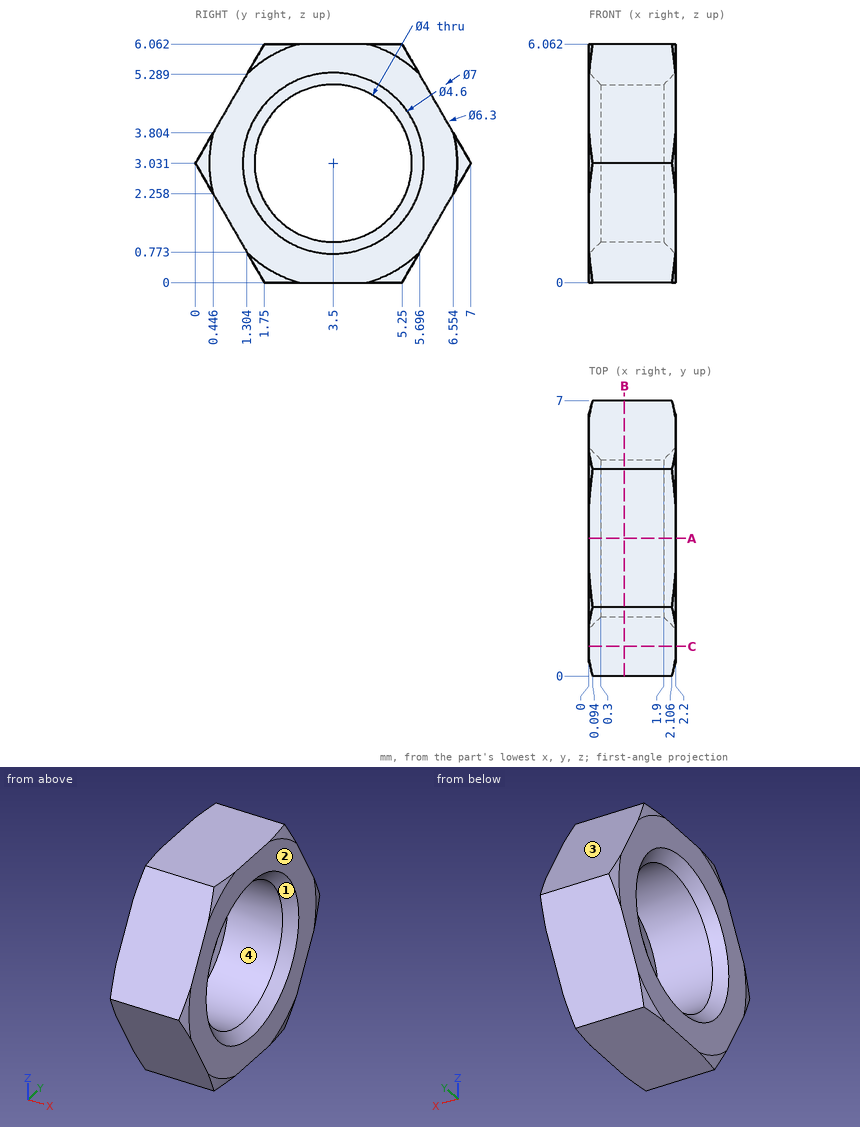
Answer from the drawing. Dimensions are ordinates in mm from the lowest x, y and z of the part. Give positions to 0.01 mm unless a question says otherwise; leave off trailing zeros. Write each loop counter-clockwise with the first axis right and the second up, starting at its lowest first coordinate (ties: lowest second). Pieces come first, ordered by that corner, then holes. Notation, with made-up numbers: M 58.25,50 L 86.25,50 A9 ccw 86.25,63 Z; hole C -9.5,65.25 d5. An arc over 180 degrees is marked long. Answer as CSV lines item,"result".
Q1. Given P1, Ø1.5, axis at y = 1, z = 3.5, coming from the -X side, flat-ended and moving along its own axis, determine where the tip first touches the part or whether it passes through.
A:
P1,"stops at x = 0"
Q2. The mould has two halves that part along Y. Classify the marked faces 1, 2, 3 and 4: +Y half, -Y half, draft (parallel to the pull), parting line (faces both ways), or undercut.
A:
face 1,"undercut"
face 2,"draft"
face 3,"+Y half"
face 4,"undercut"
Q3. A cutting plane is placed at B-B on x = 0.9. Write down the section's boundary in (y, z).
A:
outline,"M 0,3.03 L 1.75,0 L 5.25,0 L 7,3.03 L 5.25,6.06 L 1.75,6.06 Z; hole C 3.5,3.03 d4"
Q4. Find the intervals of material crossed by probe 1 along Z at (x, y) = (1.1, 3.5); probe 2 along Y at (x, z) = (1.7, 4.5); probe 3 along Y at (x, z) = (0.45, 3.5) (1 decimal), in increasing order. Write a range as [from, to].
A:
probe 1,"z = [0, 1.03], [5.03, 6.06]"
probe 2,"y = [0.85, 2.14], [4.86, 6.15]"
probe 3,"y = [0.3, 1.6], [5.4, 6.7]"
Q5. A cutting plane is placed at A-A on y = 3.5. Write down the section's boundary in (x, z).
A:
outline,"M 0,0 L 2.2,0 L 2.2,0.73 L 1.9,1.03 L 0.3,1.03 L 0,0.73 Z; M 0,5.33 L 0.3,5.03 L 1.9,5.03 L 2.2,5.33 L 2.2,6.06 L 0,6.06 Z"
Q6. A cutting plane is placed at C-C on y = 0.75. Write down the section's boundary in (x, z).
A:
outline,"M 0,1.73 L 2.2,1.73 L 2.2,4.33 L 0,4.33 Z"
